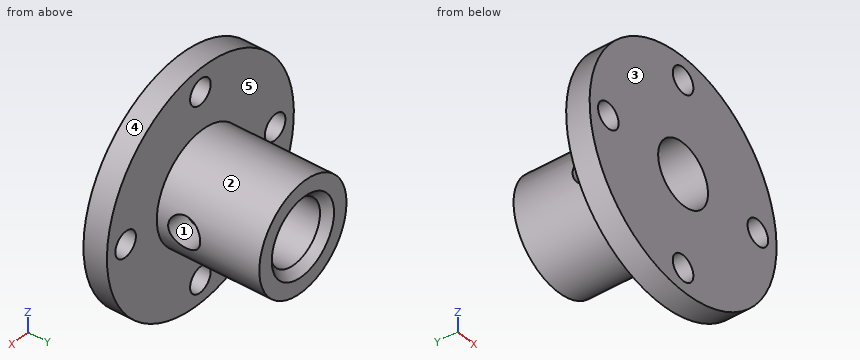
from build123d import *

# Parameters (mm, degrees)
SKETCH_1_R               = 15
SKETCH_1_R_2             = 4
EXTRUDE_1_DEPTH          = 3
SKETCH_2_R               = 7
SKETCH_2_R_2             = 4
EXTRUDE_2_DEPTH          = 13.1
CUT_EXTRUDE_1_DEPTH      = 27.630996977
CUT_EXTRUDE_1_DEPTH_BACK = 10
SKETCH_5_R               = 2.05
SKETCH_7_R               = 1.65
CUT_EXTRUDE_3_DEPTH      = 4
CHAMFER_1_SIZE           = 1


with BuildPart() as part:
    # 草图1 → 凸台-拉伸1 (new body)
    with BuildSketch(Plane(origin=(0, 0, 0), x_dir=(1, 0, 0), z_dir=(0, 1, 0))):
        with Locations(Location((0, 0, 0), (0, 0, 270))):
            Circle(SKETCH_1_R)
        with Locations(Location((0, 0, 0), (0, 0, 270))):
            Circle(SKETCH_1_R_2, mode=Mode.SUBTRACT)
    extrude(amount=EXTRUDE_1_DEPTH)

    # 草图2 → 凸台-拉伸2 (add)
    with BuildSketch(Plane(origin=(0, 3, 0), x_dir=(1, 0, 0), z_dir=(0, 1, 0))):
        with Locations(Location((0, 0, 0), (0, 0, 180))):
            Circle(SKETCH_2_R)
        with Locations(Location((0, 0, 0), (0, 0, 180))):
            Circle(SKETCH_2_R_2, mode=Mode.SUBTRACT)
    extrude(amount=EXTRUDE_2_DEPTH)

    # 草图5 → 切除-拉伸1 (cut, two sides: drawn at the far end of the back side and taken through both)
    with BuildSketch(Plane.ZY.offset(-CUT_EXTRUDE_1_DEPTH_BACK)):
        with Locations((0, 6.5)):
            Circle(SKETCH_5_R)
    extrude(amount=CUT_EXTRUDE_1_DEPTH + CUT_EXTRUDE_1_DEPTH_BACK, mode=Mode.SUBTRACT)

    # 草图7 → 切除-拉伸3 (cut)
    with BuildSketch(Plane(origin=(0, 3, 0), x_dir=(1, 0, 0), z_dir=(0, 1, 0))):
        with Locations(Location((12, 0, 0), (0, 0, 270))):
            Circle(SKETCH_7_R)
        with Locations(Location((0, -12, 0), (0, 0, 270))):
            Circle(SKETCH_7_R)
        with Locations(Location((-12, 0, 0), (0, 0, 270))):
            Circle(SKETCH_7_R)
        with Locations(Location((0, 12, 0), (0, 0, 270))):
            Circle(SKETCH_7_R)
    extrude(amount=-CUT_EXTRUDE_3_DEPTH, mode=Mode.SUBTRACT)

    # 倒角1
    # the kernel refuses this chamfer: 1 mm, written as the material it takes off along each edge
    with BuildSketch(Plane(origin=(0, 16.1, 0), x_dir=(-1, 0, 0), z_dir=(0, 0, -1))) as chamfer_1_piece_1:
        Polygon((4, -CHAMFER_1_SIZE), (4 + CHAMFER_1_SIZE, 0), (4, 0), align=None)
    revolve(axis=Axis((0, 16.1, 0), (0, 1, 0)), mode=Mode.SUBTRACT)


solid = part.part
Geometry check sheet. Reference: the model listing, model coordinates, mm. Face numbers are marked on the shaded views. A direction names the side the tool comes from. Coordinates: 2 decimals unless noted, no trailing zeros. Order: outer loops, then holes, each group sorted by start corner. A loop starts at its lowest first (then second) coordinate and runs counter-clockwise, first axis right, second up. Notation, with made-up numbers: (-35.5, 88.25) - (-23.5, 88.25) arc R19 ccw to (-23.5, 101.25) - close; hole circle Ø7 at (41, 26.5). An arc over 180 degrees is marked (long way). Answer in a Markdown table with one row per item. Add a question column.
1) Release check for a two-part mould opening along Z. For the marked faces 1, 2 and 3 record: +Z half, -Z half, draft (parallel to the pull), parting line (faces both ways), or undercut.
2) Gauge pin test, flat ends, axial feed: P1, Ø2.5, axis at y = 6.5, z = 0, coming from the -X side; P2, Ø4, axis at x = 0, z = -12, coming from the +Y side; P3, Ø5, axis at x = 1, y = 8, coming from the +Z side; P4, Ø5, axis at y = 2.5, z = 4, coming from the +X side. Record the tip position at first contact, or that the pin passes through.
3) Cross-section at C-C, the plane z = 0. State how many separate pieces and enclosed holes the cut face has, then the cut area to 3 significant figures.
4) Material ranges on line 1 along X through (y, z) = (2.3, 0); line 2 along Z through (x, y) = (-0.25, 4.25); line 3 along X through (y, z) = (11.75, 0), recorded low to high. Write a range as [from, to].
5) Cross-section at B-B, the plane y = 7.75. Record the cut outline in (x, z).
6) Set-up check for the marked faces 4 and 5: record each of +Z, -Z, +X, -X, +Y, -Y from which the full face is reachable in a straight line by a thin tool's end or side.
7) Cross-section at D-D, the plane x = 0. Record the cut outline in (y, z).
8) Cross-section at A-A, the plane x = 12. Record the cut outline in (y, z), then the cut area to 3 significant figures.
Check result:
| question | item | result |
|---|---|---|
| 1 | face 1 | undercut |
| 1 | face 2 | parting line |
| 1 | face 3 | draft |
| 2 | P1 | passes through |
| 2 | P2 | stops at y = 3 |
| 2 | P3 | stops at z = 7 |
| 2 | P4 | stops at x = 14.92 |
| 3 | separate pieces | 6 |
| 3 | enclosed holes | 0 |
| 3 | area | 99.2 mm² |
| 4 | line 1 | x = [-15, -13.65], [-10.35, -4], [4, 10.35], [13.65, 15] |
| 4 | line 2 | z = [-7, -3.99], [3.99, 7] |
| 4 | line 3 | x = [-7, -4], [4, 7] |
| 5 | outline | (-6.81, -1.62) arc R7 ccw to (6.81, -1.62) - (3.66, -1.62) arc R4 cw to (-3.66, -1.62) - close; (-6.81, 1.62) - (-3.66, 1.62) arc R4 cw to (3.66, 1.62) - (6.81, 1.62) arc R7 ccw to start |
| 6 | face 4 | +Y, -Y |
| 6 | face 5 | +Y |
| 7 | outline | (0, -15) - (3, -15) - (3, -13.65) - (0, -13.65) - close; (0, -10.35) - (3, -10.35) - (3, -7) - (16.1, -7) - (16.1, -5) - (15.1, -4) - (0, -4) - close; (0, 4) - (15.1, 4) - (16.1, 5) - (16.1, 7) - (3, 7) - (3, 10.35) - (0, 10.35) - close; (0, 13.65) - (3, 13.65) - (3, 15) - (0, 15) - close |
| 8 | outline | (0, -9) - (3, -9) - (3, -1.65) - (0, -1.65) - close; (0, 1.65) - (3, 1.65) - (3, 9) - (0, 9) - close |
| 8 | area | 44.1 mm² |
